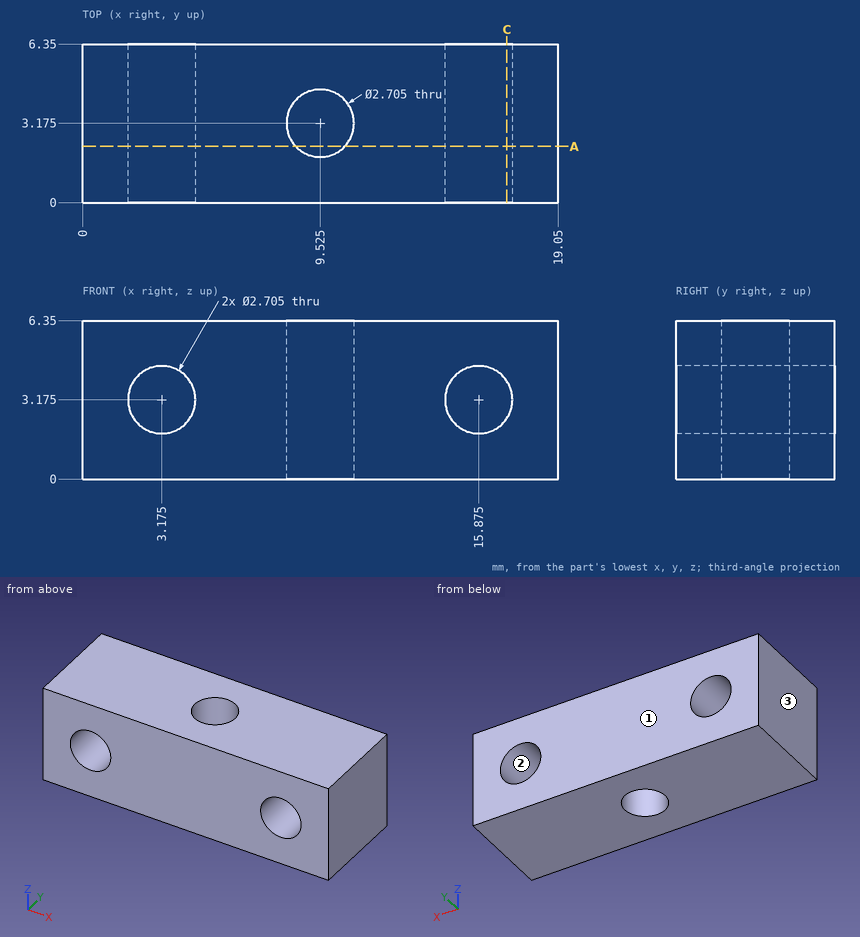
For this review, use the dimensioned drawing (mm, ordinates from the lowest corner) and the shaded views. Round coordinates to 2 decimals unless told otherwise and drop trailing zeros. Write each loop counter-clockwise with the first axis right and the second up, starting at its lowest first coordinate (ties: lowest second). Pieces come first, ordered by that corner, then holes. Notation, with made-up numbers: (-32, 86.25) -> (-2, 86.25) arc R15 ccw to (-2, 107.25) -> close; hole circle Ø2 at (-1, 47). An arc over 180 degrees is marked (long way). Use CSV: the item, a comma, the result in double quotes.
Q1. Consider section A-A (y = 2.25). State how many separate pieces and enclosed holes the cut face has.
Checks:
separate pieces,"2"
enclosed holes,"2"
Q2. Mouldability with a two-part tool opening along X and no side actions: class the marked faces 1, 2 and 3 as released by +X, released by -X, zero draft, split by the parting line, or undercut.
Checks:
face 1,"zero draft"
face 2,"undercut"
face 3,"released by -X"
Q3. For pin 1 Ø2.5 at (x, z) = (3.175, 3.175) entering from +Y, flat-tipped, find the tip position at first contact; note if it passes through.
Checks:
pin 1,"through"
Q4. To check wall thickness, follow probe 1 along X at (y, z) = (3, 3.25); probe 2 along X at (y, z) = (1.25, 2.5); probe 3 along X at (y, z) = (0.5, 4.25). State the ranges of each line that lie inside material, in increasing order. Write a range as [from, to].
Checks:
probe 1,"[0, 1.82], [4.53, 8.18], [10.87, 14.52], [17.23, 19.05]"
probe 2,"[0, 2], [4.35, 14.7], [17.05, 19.05]"
probe 3,"[0, 2.35], [4, 15.05], [16.7, 19.05]"
Q5. Consider section C-C (x = 17). Give the boundary of the cut face in (y, z).
Checks:
outline,"(0, 0) -> (6.35, 0) -> (6.35, 2.42) -> (0, 2.42) -> close; (0, 3.93) -> (6.35, 3.93) -> (6.35, 6.35) -> (0, 6.35) -> close"
